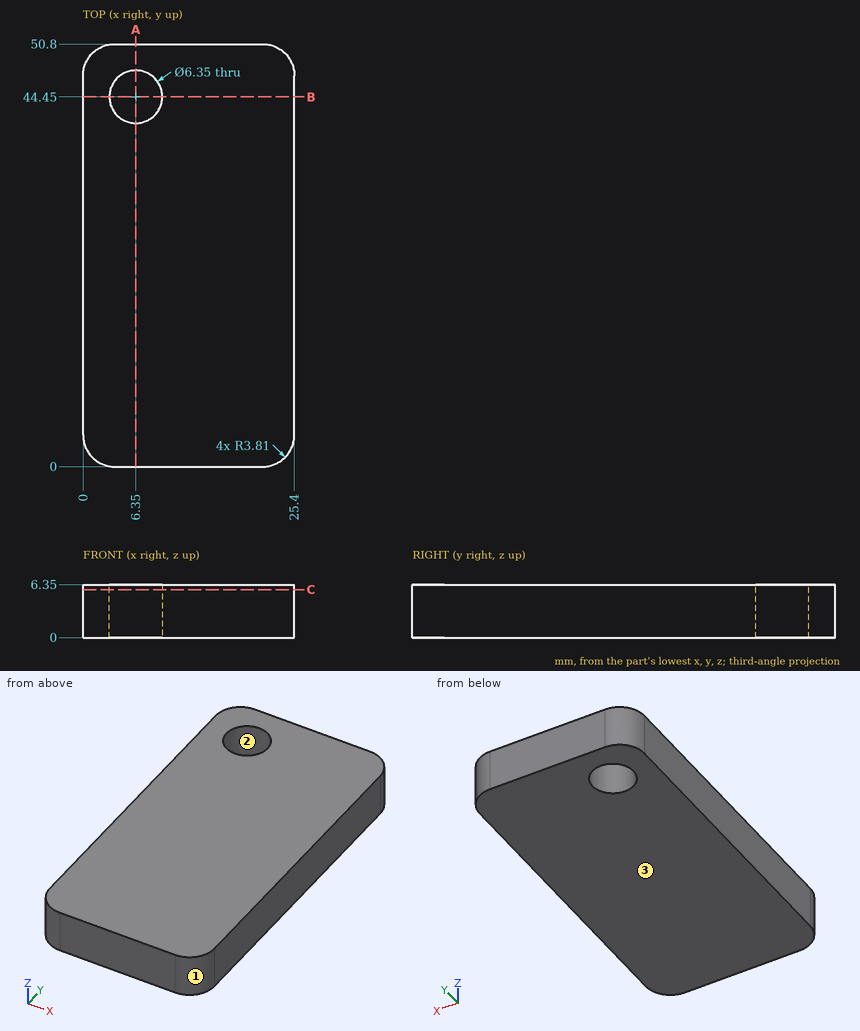
The drawing under review shows one solid part. Ordinate dimensions are in mm from its lowest x, y, z. Give positions to 0.01 mm unless a question says otherwise; leave off trailing zeros. Order: outer loops, then holes, each group sorted by start corner. A loop starts at its lowest first (then second) coordinate and runs counter-clockwise, first axis right, second up. Notation, with made-up numbers: M -0.75,-5 L 10.25,-5 A6 ccw 10.25,-1 Z; hole C 17.25,-4.75 d7. An arc over 180 degrees is marked long. Answer in a Markdown table with one row per item. Add a question column.
1. Add section B-B on y = 44.45. State the section outline as (x, z) points (3 decimals), plus the area to 3 significant figures.
2. To check wall thickness, follow line 1 along Y through (x, z) = (4.5, 6.25); line 2 along Y through (x, z) = (21.75, 2.5); line 3 along X through (y, z) = (45.5, 2.5). State the ranges of each line that lie inside material, in increasing order.
3. Mouldability with a two-part tool opening along Y and no side actions: class the marked faces 1, 2 and 3 as released by +Y, released by -Y, zero draft, split by the parting line, or undercut.
4. Add section C-C on z = 5.75. State the section outline as (x, y) points (3 decimals), plus the area to 3 significant figures.
5. For pin 1 Ø2 at (x, y) = (2.5, 27.5) entering from -Z; pin 2 Ø4 at (x, y) = (6.35, 44.45) entering from +Z, all flat-tipped, find the tip position at first contact; note any pin that passes through.
6. Add section A-A on x = 6.35. State the section outline as (y, z) points (3 decimals).
The answers:
| question | item | result |
|---|---|---|
| 1 | outline | M 0,0 L 3.175,0 L 3.175,6.35 L 0,6.35 Z; M 9.525,0 L 25.4,0 L 25.4,6.35 L 9.525,6.35 Z |
| 1 | area | 121 mm2 |
| 2 | line 1 | 0 to 41.87, 47.03 to 50.8 |
| 2 | line 2 | 0 to 50.8 |
| 2 | line 3 | 0 to 3.35, 9.35 to 25.4 |
| 3 | face 1 | released by -Y |
| 3 | face 2 | undercut |
| 3 | face 3 | zero draft |
| 4 | outline | M 0,3.81 A3.81 ccw 3.81,0 L 21.59,0 A3.81 ccw 25.4,3.81 L 25.4,46.99 A3.81 ccw 21.59,50.8 L 3.81,50.8 A3.81 ccw 0,46.99 Z; hole C 6.35,44.45 d6.35 |
| 4 | area | 1,250 mm2 |
| 5 | pin 1 | z = 0 |
| 5 | pin 2 | through |
| 6 | outline | M 0,0 L 41.275,0 L 41.275,6.35 L 0,6.35 Z; M 47.625,0 L 50.8,0 L 50.8,6.35 L 47.625,6.35 Z |
